```python
from build123d import *

# Parameters (mm, degrees)
SKETCH_1_W            = 20
SKETCH_1_H            = 20
BASEBOX_DEPTH         = 10
SKETCH_2_R            = 1
BOSSSEED_DEPTH        = 2
CIRCULARPATTERN_COUNT = 4
CIRCULARPATTERN_ANGLE = 90


with BuildPart() as part:
    # 草图1 → BaseBox (new body)
    with BuildSketch(Plane.XY):
        with Locations((10, 10)):
            Rectangle(SKETCH_1_W, SKETCH_1_H)
    extrude(amount=BASEBOX_DEPTH)

    # 草图2 → BossSeed (add)
    with BuildSketch(Plane.XY.offset(10)):
        with Locations((2, 2)):
            Circle(SKETCH_2_R)
    bossseed = extrude(amount=BOSSSEED_DEPTH)

    # CircularPattern: BossSeed ×4 about axis
    circularpattern_axis = Axis((0, 0, 0), (0, 0, -1))
    for i in range(1, CIRCULARPATTERN_COUNT):
        add(bossseed.rotate(circularpattern_axis, i * CIRCULARPATTERN_ANGLE / (CIRCULARPATTERN_COUNT - 1)))


solid = part.part
```
Design review of the part built by this model. Coordinates are the model's own, in mm. A direction names the side the tool comes from. Round coordinates to 2 decimals unless told otherwise and drop trailing zeros. Write each loop counter-clockwise with the first axis right and the second up, starting at its lowest first coordinate (ties: lowest second). Pieces come first, ordered by that corner, then holes. Notation, with made-up numbers: (-16.75, 46) -> (30.25, 46) arc R31 cw to (30.25, 79) -> close; hole circle Ø9 at (-25.5, 82). An arc over 180 degrees is marked (long way). Answer in a Markdown table with one row per item.
Q1. For faces 1 (the face through (2, -1, 10)), 2 (the face through (10, 10, 0)), list the 3-axis set-ups (+Z, -Z, +X, -X, +Y, -Y) from which the entire face can be reached by the end or side of a thin tool; tool diameter is ignored.
The answers:
| item | result |
|---|---|
| face 1 | -Z, +X, -X, -Y |
| face 2 | -Z, +X, -X, +Y, -Y |
Q2. Clearance check with flat-ended pins moving along their axes: pin 1 Ø1 at (x, y) = (17, 0.5) entering from +Z; pin 2 Ø5 at (x, z) = (10.5, 9) entering from -Y. State where each tip first meets the part, or that it passes through.
The answers:
| item | result |
|---|---|
| pin 1 | z = 10 |
| pin 2 | y = 0 |
Q3. Take a section at B-B, the plane z = 7. State the section outline as (x, y) points.
The answers:
| item | result |
|---|---|
| outline | (0, 0) -> (20, 0) -> (20, 20) -> (0, 20) -> close |
Q4. Draft analysis for pull direction Y (two halves, no side actions). For faces 3 (the face through (1.764, 0.481, 10.986)), 4 (the face through (10, 20, 5)), 5 (the face through (2.4, 0, 12)), state which applies: +Y half, -Y half, draft (parallel to the pull), parting line (faces both ways), or undercut.
The answers:
| item | result |
|---|---|
| face 3 | undercut |
| face 4 | +Y half |
| face 5 | draft |
Q5. To check wall thickness, follow L1, parallel to Y at x = 1.25, z = 3.75; L2, parallel to Z at x = 12.75, y = 1.5; L3, parallel to X at y = -0.5, z = 11.75. State the ranges of each line that lie inside material, in increasing order. Write a range as [from, to].
The answers:
| item | result |
|---|---|
| L1 | [0, 20] |
| L2 | [0, 10] |
| L3 | [1.76, 3.7] |
Q6. Take a section at A-A, the plane y = 2. State the section outline as (x, z) points, then the cut area to 3 significant figures.
The answers:
| item | result |
|---|---|
| outline | (0, 0) -> (20, 0) -> (20, 10) -> (3, 10) -> (3, 12) -> (1, 12) -> (1, 10) -> (0, 10) -> close |
| area | 204 mm² |
Q7. Take a section at C-C, the plane x = 12.25. State the section outline as (y, z) points.
The answers:
| item | result |
|---|---|
| outline | (0, 0) -> (20, 0) -> (20, 10) -> (0, 10) -> close |
